For this review, take the finished solid that the model builds, in its own axes (mm). Give positions to 0.01 mm unless a question says otherwise; leave off trailing zeros. Order: outer loops, then holes, each group sorted by start corner. A loop starts at its lowest first (then second) coordinate and runs counter-clockwise, first axis right, second up. Notation, with made-up numbers: (67.5, 31) - (87.5, 31) arc R20 cw to (87.5, 55) - close; hole circle Ø3 at (-30.75, 77.5). An arc over 180 degrees is marked (long way). One line per item, written item: value.
```python
from build123d import *

# Parameters (mm, degrees)
F1_DEPTH = 12.7


with BuildPart() as f1:
    # F0 (on Right) → F1 (new body)
    with BuildSketch(Plane.YZ):
        with BuildLine():
            ThreePointArc((-274.750656, 90.78483), (-276.709945, 95.081547), (-281.093691, 96.8375))
            Line((-281.093691, 96.8375), (-283.102754, 96.8375))
            ThreePointArc((-283.102754, 96.8375), (-286.627633, 95.76933), (-288.966632, 92.924185))
            add(Edge.make_bspline(
                [(-288.966632, 92.924185), (-302.669456, 59.948361), (-302.669456, 57.526639), (-288.966632, 24.550815)],
                knots=[2.702454, 2.702454, 2.702454, 2.702454, 73.497546, 73.497546, 73.497546, 73.497546], degree=3))
            ThreePointArc((-288.966632, 24.550815), (-286.627633, 21.70567), (-283.102754, 20.6375))
            Line((-283.102754, 20.6375), (-281.093691, 20.6375))
            ThreePointArc((-281.093691, 20.6375), (-276.709945, 22.393453), (-274.750656, 26.69017))
            Line((-274.750656, 26.69017), (-273.91468, 44.524332))
            ThreePointArc((-273.91468, 44.524332), (-273.424857, 45.598512), (-272.328921, 46.0375))
            Line((-272.328921, 46.0375), (-254, 46.0375))
            ThreePointArc((-254, 46.0375), (-252.877468, 45.572532), (-252.4125, 44.45))
            Line((-252.4125, 44.45), (-252.4125, -44.45))
            ThreePointArc((-252.4125, -44.45), (-252.877468, -45.572532), (-254, -46.0375))
            Line((-254, -46.0375), (-272.328921, -46.0375))
            ThreePointArc((-272.328921, -46.0375), (-273.424857, -45.598512), (-273.91468, -44.524332))
            Line((-273.91468, -44.524332), (-274.750656, -26.69017))
            ThreePointArc((-274.750656, -26.69017), (-276.709945, -22.393453), (-281.093691, -20.6375))
            Line((-281.093691, -20.6375), (-283.102754, -20.6375))
            ThreePointArc((-283.102754, -20.6375), (-286.627633, -21.70567), (-288.966632, -24.550815))
            add(Edge.make_bspline(
                [(-288.966632, -92.924185), (-302.669456, -59.948361), (-302.669456, -57.526639), (-288.966632, -24.550815)],
                knots=[2.702454, 2.702454, 2.702454, 2.702454, 73.497546, 73.497546, 73.497546, 73.497546], degree=3))
            ThreePointArc((-288.966632, -92.924185), (-286.627633, -95.76933), (-283.102754, -96.8375))
            Line((-283.102754, -96.8375), (-281.093691, -96.8375))
            ThreePointArc((-281.093691, -96.8375), (-276.709945, -95.081547), (-274.750656, -90.78483))
            Line((-274.750656, -90.78483), (-273.91468, -72.950668))
            ThreePointArc((-273.91468, -72.950668), (-273.424857, -71.876488), (-272.328921, -71.4375))
            Line((-272.328921, -71.4375), (-254, -71.4375))
            ThreePointArc((-254, -71.4375), (-252.877468, -71.902468), (-252.4125, -73.025))
            Line((-252.4125, -73.025), (-252.4125, -122.2375))
            Line((-252.4125, -122.2375), (227.0125, -122.2375))
            Line((227.0125, -122.2375), (227.0125, -73.025))
            ThreePointArc((227.0125, -73.025), (227.477468, -71.902468), (228.6, -71.4375))
            Line((228.6, -71.4375), (246.928921, -71.4375))
            ThreePointArc((246.928921, -71.4375), (248.024857, -71.876488), (248.51468, -72.950668))
            Line((248.51468, -72.950668), (249.350656, -90.78483))
            ThreePointArc((249.350656, -90.78483), (251.309945, -95.081547), (255.693691, -96.8375))
            Line((255.693691, -96.8375), (257.702754, -96.8375))
            ThreePointArc((257.702754, -96.8375), (261.227633, -95.76933), (263.566632, -92.924185))
            add(Edge.make_bspline(
                [(263.566632, -92.924185), (277.269456, -59.948361), (277.269456, -57.526639), (263.566632, -24.550815)],
                knots=[2.702454, 2.702454, 2.702454, 2.702454, 73.497546, 73.497546, 73.497546, 73.497546], degree=3))
            ThreePointArc((263.566632, -24.550815), (261.227633, -21.70567), (257.702754, -20.6375))
            Line((257.702754, -20.6375), (255.693691, -20.6375))
            ThreePointArc((255.693691, -20.6375), (251.309945, -22.393453), (249.350656, -26.69017))
            Line((249.350656, -26.69017), (248.51468, -44.524332))
            ThreePointArc((248.51468, -44.524332), (248.024857, -45.598512), (246.928921, -46.0375))
            Line((246.928921, -46.0375), (228.6, -46.0375))
            ThreePointArc((228.6, -46.0375), (227.477468, -45.572532), (227.0125, -44.45))
            Line((227.0125, -44.45), (227.0125, 44.45))
            ThreePointArc((227.0125, 44.45), (227.477468, 45.572532), (228.6, 46.0375))
            Line((228.6, 46.0375), (246.928921, 46.0375))
            ThreePointArc((246.928921, 46.0375), (248.024857, 45.598512), (248.51468, 44.524332))
            Line((248.51468, 44.524332), (249.350656, 26.69017))
            ThreePointArc((249.350656, 26.69017), (251.309945, 22.393453), (255.693691, 20.6375))
            Line((255.693691, 20.6375), (257.702754, 20.6375))
            ThreePointArc((257.702754, 20.6375), (261.227633, 21.70567), (263.566632, 24.550815))
            add(Edge.make_bspline(
                [(263.566632, 92.924185), (277.269456, 59.948361), (277.269456, 57.526639), (263.566632, 24.550815)],
                knots=[2.702454, 2.702454, 2.702454, 2.702454, 73.497546, 73.497546, 73.497546, 73.497546], degree=3))
            ThreePointArc((263.566632, 92.924185), (261.227633, 95.76933), (257.702754, 96.8375))
            Line((257.702754, 96.8375), (255.693691, 96.8375))
            ThreePointArc((255.693691, 96.8375), (251.309945, 95.081547), (249.350656, 90.78483))
            Line((249.350656, 90.78483), (248.51468, 72.950668))
            ThreePointArc((248.51468, 72.950668), (248.024857, 71.876488), (246.928921, 71.4375))
            Line((246.928921, 71.4375), (228.6, 71.4375))
            ThreePointArc((228.6, 71.4375), (227.477468, 71.902468), (227.0125, 73.025))
            Line((227.0125, 73.025), (227.0125, 122.2375))
            Line((227.0125, 122.2375), (-252.4125, 122.2375))
            Line((-252.4125, 122.2375), (-252.4125, 73.025))
            ThreePointArc((-252.4125, 73.025), (-252.877468, 71.902468), (-254, 71.4375))
            Line((-254, 71.4375), (-272.328921, 71.4375))
            ThreePointArc((-272.328921, 71.4375), (-273.424857, 71.876488), (-273.91468, 72.950668))
            Line((-273.91468, 72.950668), (-274.750656, 90.78483))
        make_face()
    extrude(amount=F1_DEPTH)


solid = f1.part
```
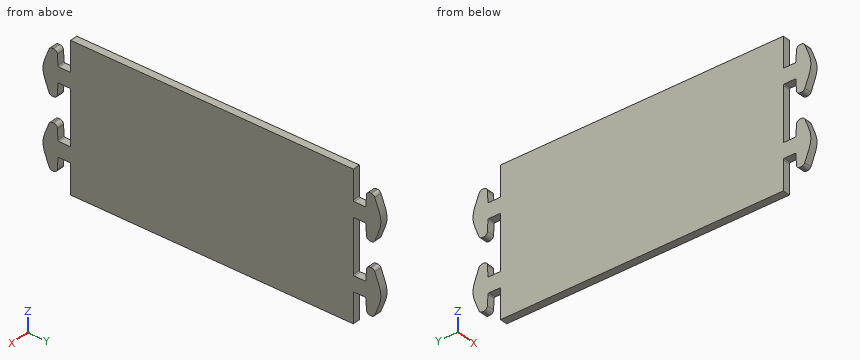
(1) Wall thickness on line 1 (Y direction, x = 2, z = 22); line 2 (Y direction, x = 11, z = 94.5); line 3 (Y direction, x = 6, z = 104): over which ranges is each line inside the solid? List them lowest first. Write a range as from..to.
Answers below:
line 1: y = -287.03..-277.16, -252.41..227.01, 251.76..261.63
line 2: y = -288.02..-276.17, -252.41..227.01, 250.77..262.62
line 3: y = -252.41..227.01
(2) For P1, Ø1, axis at x = 3.5, y = -282.5, coming from the -Z side; P2, Ø3, axis at x = 9.5, z = -12, coming from the +Y side; P3, Ø1, axis at x = 5, y = -282, coming from the +Z side, all flat-tipped, find the tip position at first contact; note any pin that passes through.
Answers below:
P1: stops at z = -96.84
P2: stops at y = 227.01
P3: stops at z = 96.84
(3) Take a section at A-A (z = 2). Write out the cut boundary in (x, y), then the cut area to 3 significant figures.
Answers below:
outline: (0, -252.41) - (12.7, -252.41) - (12.7, 227.01) - (0, 227.01) - close
area: 6,090 mm^2
